from build123d import *

# Parameters (mm, degrees)
SKETCH1_R           = 13.4
BOSS_EXTRUDE1_DEPTH = 30
BOSS_EXTRUDE2_DEPTH = 34.8


with BuildPart() as part:
    # Sketch1 → Boss-Extrude1 (new body)
    with BuildSketch(Plane(origin=(0, 0, 0), x_dir=(1, 0, 0), z_dir=(0, 1, 0))):
        Polygon((-17.4, 17.4), (17.4, 17.4), (82.6, 17.4), (82.6, 13.4), (17.4, 13.4), (17.4, -17.4), (-17.4, -17.4), align=None)
        with Locations(Location((0, 0, 0), (0, 0, 270))):
            Circle(SKETCH1_R, mode=Mode.SUBTRACT)
    extrude(amount=BOSS_EXTRUDE1_DEPTH)

    # Sketch3 → Boss-Extrude2 (add)
    with BuildSketch(Plane.ZY.offset(17.4)):
        with BuildLine():
            Line((-17.4, 0), (-32.4, 0))
            Line((-32.4, 0), (-32.4, 3))
            ThreePointArc((-32.4, 3), (-27.598787547, 3.605237022), (-24.805858924, 7.557135626))
            Line((-24.805858924, 7.557135626), (-17.4, 7.557135626))
            Line((-17.4, 7.557135626), (-17.4, 0))
        make_face()
        with BuildLine():
            Line((-32.4, 14.5), (-32.4, 17.5))
            Line((-32.4, 17.5), (-17.4, 17.5))
            Line((-17.4, 17.5), (-17.4, 10.557135626))
            Line((-17.4, 10.557135626), (-24.964700082, 10.557135626))
            ThreePointArc((-24.964700082, 10.557135626), (-27.875124937, 14.050801443), (-32.4, 14.5))
        make_face()
    extrude(amount=-BOSS_EXTRUDE2_DEPTH)


solid = part.part
Verification items for the finished model (mm, model axes). A direction names the side the tool comes from. Give positions to 0.01 mm unless a question says otherwise; leave off trailing zeros. Write each loop counter-clockwise with the first axis right and the second up, starting at its lowest first coordinate (ties: lowest second). Pieces come first, ordered by that corner, then holes.
(1) Gauge pin test, flat ends, axial feed: pin 1 (2 mm diameter, centred on x = 48.5, y = 5.5, fed in from -Z); pin 2 (4.5 mm diameter, centred on x = 1, z = -24, fed in from +Y); pin 3 (2 mm diameter, centred on y = 15.5, z = -10, fed in from +X); pin 4 (24 mm diameter, centred on x = 0, z = 0, fed in from +Y). Record the tip position at first contact, or that the pin passes through.
(2) Cross-section at D-D (z = 0). Enter the section's corners in (x, y), plus the area to 3 significant figures.
(3) Material ranges on line 1 (X direction, y = 6.25, z = 0); line 2 (Z direction, x = -11, y = 23.75); line 3 (X direction, y = 6, z = -5), recorded low to high.
(4) Cross-section at A-A (x = 0). Enter the section's corners in (y, z), plus the area to 3 significant figures.
(5) Access from +Z, -Z, +X, -X, +Y, -Y to the whole of each face (thin tool, end or side, straight path). Record for faces 4 (the face through (17.4, 3, -23)), 5 (the face through (0, 17.5, -25)), 6 (the face through (0, 10.557, -21)), 7 (the face through (50, 15, -13.4)).
(6) Mould release check, pull along Z, two halves, no side actions. Record for faces 1 (the face through (0, 16, -32.4)), 2 (the face through (82.6, 15, -15)), 3 (the face through (-0.24, 3.57, -27.66)): +Z half, -Z half, draft (parallel to the pull), parting line (faces both ways), or undercut.
(7) Cross-section at C-C (y = 24.5). Enter the section's corners in (x, z), plus the area to 3 significant figures.
(8) Cross-section at B-B (z = -20). Enter the section's corners in (x, y).
Worked out:
1. pin 1: stops at z = -17.4
1. pin 2: stops at y = 17.5
1. pin 3: stops at x = 17.4
1. pin 4: passes through
2. outline: (-17.4, 0) - (-13.4, 0) - (-13.4, 30) - (-17.4, 30) - close; (13.4, 0) - (17.4, 0) - (17.4, 30) - (13.4, 30) - close
2. area: 240 mm2
3. line 1: x = -17.4 to -13.4, 13.4 to 17.4
3. line 2: z = -17.4 to -7.65, 7.65 to 17.4
3. line 3: x = -17.4 to -12.43, 12.43 to 17.4
4. outline: (0, -32.4) - (3, -32.4) arc R6 cw to (7.56, -24.81) - (7.56, -17.4) - (10.56, -17.4) - (10.56, -24.96) arc R6 cw to (14.5, -32.4) - (17.5, -32.4) - (17.5, -17.4) - (30, -17.4) - (30, -13.4) - (0, -13.4) - close; (0, 13.4) - (30, 13.4) - (30, 17.4) - (0, 17.4) - close
4. area: 404 mm2
5. face 4: -Z, +X, +Y, -Y
5. face 5: -Z, +X, -X, +Y
5. face 6: -Z, +X, -X
5. face 7: +Z, +X, +Y, -Y
6. face 1: -Z half
6. face 2: draft
6. face 3: undercut
7. outline: (-17.4, -17.4) - (82.6, -17.4) - (82.6, -13.4) - (17.4, -13.4) - (17.4, 17.4) - (-17.4, 17.4) - close; hole circle Ø26.8 at (0, 0)
7. area: 908 mm2
8. outline: (-17.4, 0) - (17.4, 0) - (17.4, 7.56) - (-17.4, 7.56) - close; (-17.4, 10.56) - (17.4, 10.56) - (17.4, 17.5) - (-17.4, 17.5) - close
